Read the model definition and answer for the solid it produces. Units are mm, in the model's axes. A direction names the side the tool comes from. Coordinates: 2 decimals unless noted, no trailing zeros. Write each loop counter-clockwise with the first axis right and the second up, starting at its lowest first coordinate (ties: lowest second). Pieces come first, ordered by that corner, then holes. Notation, with made-up numbers: M 33,45 L 71,45 A15 ccw 71,60 Z; hole C 34.5,18 d10. An arc over 180 degrees is marked long. Use a Markdown table: item, result. Add a question column.
from build123d import *

# Parameters (mm, degrees)
SKETCH_R      = 92
SKETCH_R_2    = 90
PAD_DEPTH     = 40
SKETCH001_R   = 130
SKETCH001_R_2 = 90
PAD001_DEPTH  = 2


with BuildPart() as part:
    # Sketch → Pad (new body)
    with BuildSketch(Plane.XY):
        Circle(SKETCH_R)
        Circle(SKETCH_R_2, mode=Mode.SUBTRACT)
    extrude(amount=PAD_DEPTH)

    # Sketch001 (on Face4 of Pad) → Pad001 (join)
    with BuildSketch(Plane.XY.offset(40)):
        with Locations((-0.139716, -0.307385)):
            Circle(SKETCH001_R)
        with Locations((-0.139716, -0.307385)):
            Circle(SKETCH001_R_2, mode=Mode.SUBTRACT)
    extrude(amount=PAD001_DEPTH)


solid = part.part
Item 1: Each of these flat-tipped pins is pushed along its axis until it touches: pin 1 (10 mm diameter, centred on x = -67.5, z = 37, fed in from -Y); pin 2 (12 mm diameter, centred on y = -68, z = 22, fed in from -X); pin 3 (4 mm diameter, centred on y = 81, z = 30, fed in from +X). Where does it stop, or does it pass through?
Item 2: For faces 4 (the flat face through (-89, -27, 40)), 5 (the flat face through (68, -61, 0)), determine the directions among +Z, -Z, +X, -X, +Y, -Y from which every point of the face is accessible in a straight line to the end or side of a thin tool.
Item 3: Determine the mould class of faces 1 (the cylindrical face through (-19.65, -88.167, 40.986)), 2 (the cylindrical face through (-28.321, -127.216, 40.986)), 3 (the flat face through (-30.8, -85.2, 42)) for opening direction Y: pulls with the +Y half, pulls with the -Y half, needs draft (parallel to the pull), parting line crosses it, or undercut.
Item 4: Consider probe 1 along Y at (x, z) = (0, 30); probe 2 along X at (y, z) = (1, 16); probe 3 along Z at (x, y) = (-56, -98.5). Determine where each line is inside the solid, lowest interval first.
Item 5: Find section A-A on y = -62. Give the vertices of the cut face in (x, z), then the cut area to 3 significant figures.
Item 6: Find section D-D on y = 110.5. Give the vertices of the cut face in (x, z), then the cut area to 3 significant figures.
Item 7: Find section C-C on z = 10.5. Give the vertices of the cut face in (x, y), then the cut area to 3 significant figures.
Item 8: Find section B-B on x = 48. Give the vertices of the cut face in (y, z).
Geometry says:
| question | item | result |
|---|---|---|
| 1 | pin 1 | stops at y = -113.82 |
| 1 | pin 2 | stops at x = -67.97 |
| 1 | pin 3 | stops at x = 47.15 |
| 2 | face 4 | -Z |
| 2 | face 5 | -Z, +X, -X, +Y, -Y |
| 3 | face 1 | undercut |
| 3 | face 2 | parting line crosses it |
| 3 | face 3 | needs draft |
| 4 | probe 1 | y = -92 to -90, 90 to 92 |
| 4 | probe 2 | x = -91.99 to -89.99, 89.99 to 91.99 |
| 4 | probe 3 | z = 40 to 42 |
| 5 | outline | M -114.57,40 L -67.97,40 L -67.97,0 L -65.24,0 L -65.24,40 L -65.67,40 L -65.67,42 L -114.57,42 Z; M 65.24,0 L 67.97,0 L 67.97,40 L 114.29,40 L 114.29,42 L 65.39,42 L 65.39,40 L 65.24,40 Z |
| 5 | area | 414 mm2 |
| 6 | outline | M -68.12,40 L 67.84,40 L 67.84,42 L -68.12,42 Z |
| 6 | area | 272 mm2 |
| 7 | outline | C 0,0 d184; hole C 0,0 d180 |
| 7 | area | 1,140 mm2 |
| 8 | outline | M -121.07,40 L -78.49,40 L -78.49,0 L -76.13,0 L -76.13,40 L -76.35,40 L -76.35,42 L -121.07,42 Z; M 75.74,40 L 76.13,40 L 76.13,0 L 78.49,0 L 78.49,40 L 120.45,40 L 120.45,42 L 75.74,42 Z |
